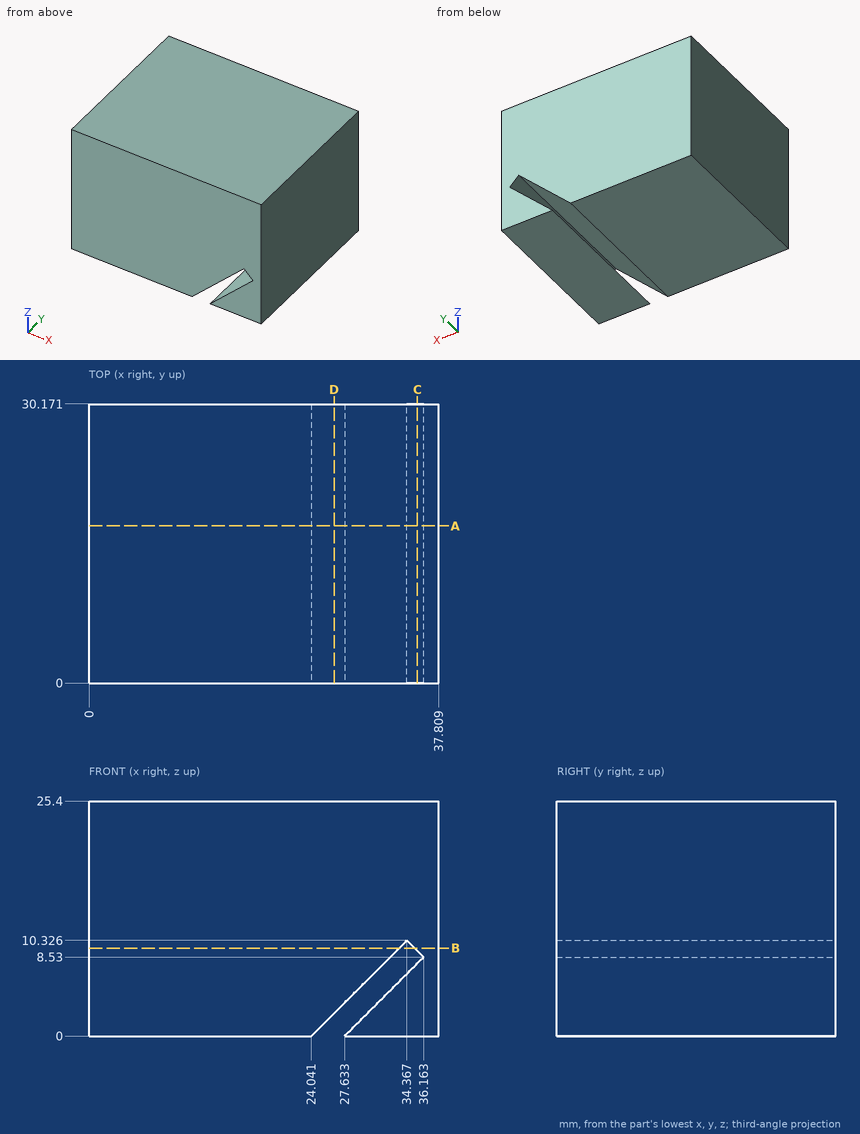
Check sheet for the drawn part. Datum: minimum x, y, z corner. Units: mm. Round coordinates to 2 decimals unless told otherwise and drop trailing zeros. Order: outer loops, then holes, each group sorted by start corner. A loop starts at its lowest first (then second) coordinate and runs counter-clockwise, first axis right, second up.
1. Go/stop test with a flat-tipped pin: P1, Ø2, axis at x = 25.5, y = 23, coming from the -Z side. Record where the tip stops, or that it passes through.
Final values:
P1: stops at z = 0.46
2. Thickness scan on L1, parallel to X at y = 14.5, z = 7.5; L2, parallel to X at y = 12, z = 9.5; L3, parallel to Z at x = 33.5, y = 4. Record the ranges inside material, lowest first.
Final values:
L1: x = 0 to 31.54, 35.13 to 37.81
L2: x = 0 to 33.54, 35.19 to 37.81
L3: z = 0 to 5.87, 9.46 to 25.4
3. Section check C-C on x = 35.5. Record the cut outline in (y, z).
Final values:
outline: (0, 0) - (30.17, 0) - (30.17, 7.87) - (0, 7.87) - close; (0, 9.19) - (30.17, 9.19) - (30.17, 25.4) - (0, 25.4) - close
4. Section check B-B on z = 9.5. Record the cut outline in (x, y).
Final values:
outline: (0, 0) - (33.54, 0) - (33.54, 30.17) - (0, 30.17) - close; (35.19, 0) - (37.81, 0) - (37.81, 30.17) - (35.19, 30.17) - close
5. Section check D-D on x = 26.5. Record the cut outline in (y, z).
Final values:
outline: (0, 2.46) - (30.17, 2.46) - (30.17, 25.4) - (0, 25.4) - close
6. Section check A-A on y = 17. Record the cut outline in (x, z).
Final values:
outline: (0, 0) - (24.04, 0) - (34.37, 10.33) - (36.16, 8.53) - (27.63, 0) - (37.81, 0) - (37.81, 25.4) - (0, 25.4) - close
